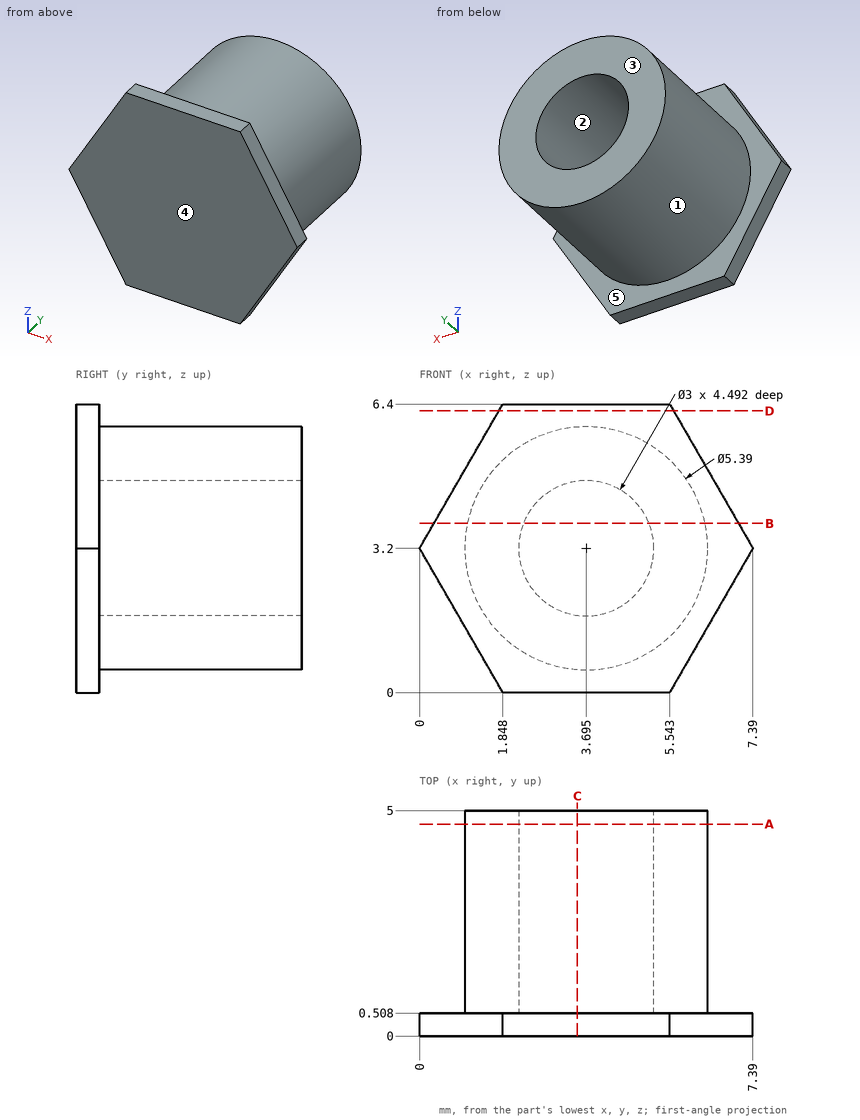
Can you work these out from the drawing? Everything is in mm from the part's minimum corner. A direction names the side the tool comes from. Round coordinates to 2 decimals unless told otherwise and drop trailing zeros. Write each loop counter-clockwise with the first axis right and the second up, starting at its lowest first coordinate (ties: lowest second). Pieces come first, ordered by that corner, then holes.
1. I need wall thicknesses on L1, parallel to Y at x = 3, z = 2; L2, parallel to Z at x = 3.5, y = 4.85; L3, parallel to X at y = 3.85, z = 3.5 (1 decimal). Which ranges of each line are inside material? Lowest first, please.
2. Suppose I cut it at C-C (x = 3.5). List the corners of the cut face in (y, z) for me.
3. Suppose I cut it at B-B (z = 3.75). List the corners of the cut face in (x, y) for me, and give its area (3 significant figures).
4. Suppose I cut it at A-A (y = 4.7). List the corners of the cut face in (x, z) for me (1 decimal).
5. Will these pins go through, and if not, where does the flat tip stop? pin 1 Ø1 at (y, z) = (3, 5) entering from +X (1 decimal); pin 2 Ø0.9 at (x, z) = (3.5, 3.5) entering from +Y.
6. Suppose I cut it at D-D (z = 6.25). List the corners of the cut face in (x, y) for me.
7. If we mould it in two halves opening along X, with no side actions, what happens to the marked faces 1, 2 and 3? For each: released by +X, released by -X, zero draft, split by the parting line, or undercut.
8. For the marked faces 4 and 5, which set-ups out of +Z, -Z, +X, -X, +Y, -Y let a thin tool reach every point of the face, with its end or its side?
Answer sheet:
1. L1: y = 0 to 0.51
1. L2: z = 0.51 to 1.71, 4.69 to 5.89
1. L3: x = 1 to 2.2, 5.2 to 6.4
2. outline: (0, 0) - (0.51, 0) - (0.51, 0.51) - (5, 0.51) - (5, 1.71) - (0.51, 1.71) - (0.51, 4.69) - (5, 4.69) - (5, 5.89) - (0.51, 5.89) - (0.51, 6.4) - (0, 6.4) - close
3. outline: (0.32, 0) - (7.07, 0) - (7.07, 0.51) - (6.33, 0.51) - (6.33, 5) - (5.09, 5) - (5.09, 0.51) - (2.3, 0.51) - (2.3, 5) - (1.06, 5) - (1.06, 0.51) - (0.32, 0.51) - close
3. area: 14.6 mm2
4. outline: circle Ø5.4 at (3.7, 3.2); hole circle Ø3 at (3.7, 3.2)
5. pin 1: stops at x = 6.1
5. pin 2: stops at y = 0.51
6. outline: (1.76, 0) - (5.63, 0) - (5.63, 0.51) - (1.76, 0.51) - close
7. face 1: split by the parting line
7. face 2: undercut
7. face 3: zero draft
8. face 4: +Z, -Z, +X, -X, -Y
8. face 5: +Y
